For this review, take the finished solid that the model builds, in its own axes (mm). A direction names the side the tool comes from. Round coordinates to 2 decimals unless told otherwise and drop trailing zeros. Loops run counter-clockwise (first coordinate to the right, second up) from the corner with the lowest first, then second, coordinate; pieces in that order, holes last. Notation, with made-up numbers: (51, 4.25) -> (85, 4.25) arc R25 cw to (85, 41.25) -> close; hole circle Ø1 at (15, 88.25). An arc over 180 degrees is marked (long way). One line per question, with ' | ' between items. Start each with the question number.
1. Consider section A-A (y = -130.5). Write out the cut boundary in (x, z), and give its area (3 significant figures).
2. Draft analysis for pull direction Z (two halves, no side actions). For faces 6 (the face through (3, -2, 10)), 7 (the face through (-3, -85, 10)), 8 (the face through (4.848, 8.746, 2.465)), 9 (the face through (0.14, -129.87, 13.09)), state which applies: pulls with the +Z half, pulls with the -Z half, needs draft (parallel to the pull), parting line crosses it, or undercut.
3. For faces 1 (the face through (0, -37, 0)), 2 (the face through (1, -15, 8)), 3 (the face through (-10, -51, 7)), 4 (the face through (5, -85, 7)), 5 (the face through (-5.047, 2, 2)), list the 3-axis set-ups (+Z, -Z, +X, -X, +Y, -Y) from which the entire face can be reached by the end or side of a thin tool; tool diameter is ignored.
4. For pin 1 Ø5.5 at (y, z) = (-200, 8) entering from -X; pin 2 Ø2.5 at (x, z) = (-1.5, 7) entering from +Y; pin 3 Ø4 at (y, z) = (-201, 9) entering from +X; pin 4 Ø2.5 at (x, y) = (0, -85) entering from +Z, all flat-tipped, find the tip position at first contact; note any pin that passes through.
5. Wall thickness on line 1 along Z through (x, y) = (-4.25, -86); line 2 along X through (y, z) = (-85, 11.15); line 3 along X through (y, z) = (-72.5, 7.5): over which ranges is each line inside the solid? List them lowest first.
6. Consider section B-B (y = -158). Write out the cut boundary in (x, z), and give its area (3 significant figures).
```python
from build123d import *

# Parameters (mm, degrees)
CROQUIS1_R              = 1.5
SALIENTE_EXTRUIR1_DEPTH = 15
CROQUIS2_W              = 5
CROQUIS2_H              = 15
CROQUIS2_H_2            = 35
CORTAR_EXTRUIR1_DEPTH   = 60
CROQUIS4_W              = 5
CROQUIS4_H              = 30
CORTAR_EXTRUIR2_DEPTH   = 15
CORTAR_EXTRUIR3_DEPTH   = 40


with BuildPart() as part:
    # Croquis1 → Saliente-Extruir1 (new body)
    with BuildSketch(Plane.XY):
        with BuildLine():
            Line((10, 0), (10, -85))
            Line((10, -85), (2.49701529, -197.5))
            Line((2.49701529, -197.5), (2.49701529, -202.5))
            Line((2.49701529, -202.5), (-2.49701529, -202.5))
            Line((-2.49701529, -202.5), (-2.49701529, -197.5))
            Line((-2.49701529, -197.5), (-10, -85))
            Line((-10, -85), (-10, 0))
            ThreePointArc((-10, 0), (0, 10), (10, 0))
        make_face()
        with Locations((0, -85)):
            Circle(CROQUIS1_R, mode=Mode.SUBTRACT)
        Circle(CROQUIS1_R, mode=Mode.SUBTRACT)
    extrude(amount=SALIENTE_EXTRUIR1_DEPTH)

    # Croquis2 → Cortar-Extruir1 (cut)
    with BuildSketch(Plane(origin=(10, 0, 0), x_dir=(0, 0, -1), z_dir=(1, 0, 0))):
        with Locations((-7.5, -7.5)):
            Rectangle(CROQUIS2_W, CROQUIS2_H)
        with Locations((-7.5, 17.5)):
            Rectangle(CROQUIS2_W, CROQUIS2_H_2)
        Polygon((-15, -85), (-10, -202.5), (-18.081893827, -208.021253548), align=None)
        Polygon((-5, -202.5), (3.081893827, -208.021253548), (0, -85), align=None)
    extrude(amount=-CORTAR_EXTRUIR1_DEPTH, mode=Mode.SUBTRACT)

    # Croquis4 → Cortar-Extruir2 (cut)
    with BuildSketch(Plane.ZY.offset(10)):
        with Locations((7.5, -85)):
            Rectangle(CROQUIS4_W, CROQUIS4_H)
    extrude(amount=-CORTAR_EXTRUIR2_DEPTH, mode=Mode.SUBTRACT)

    # Croquis5 → Cortar-Extruir3 (cut)
    with BuildSketch(Plane(origin=(0, 0, 0), x_dir=(-1, 0, 0), z_dir=(0, 0, -1))):
        with BuildLine():
            Line((20.047011477, -20), (24.874582677, -20))
            Line((24.874582677, -20), (24.874582677, 13.063406197))
            Line((24.874582677, 13.063406197), (10, 13.063406197))
            Line((10, 13.063406197), (10, 14.482732523))
            Line((10, 14.482732523), (5.047011477, 14.482732523))
            Line((5.047011477, 14.482732523), (5.047011477, -5))
            ThreePointArc((5.047011477, -5), (9.440409759, -15.606601718), (20.047011477, -20))
        make_face()
    extrude(amount=-CORTAR_EXTRUIR3_DEPTH, mode=Mode.SUBTRACT)


solid = part.part
```
Answer block:
1) outline: (-6.97, 1.94) -> (6.97, 1.94) -> (6.97, 13.06) -> (-6.97, 13.06) -> close | area: 155 mm2
2) face 6: undercut | face 7: undercut | face 8: needs draft | face 9: pulls with the +Z half
3) face 1: -Z, +X, -X, +Y, -Y | face 2: +X, -X, +Y | face 3: +Z, -Z, -X, +Y, -Y | face 4: -X | face 5: +Z, -Z, -X, +Y
4) pin 1: stops at x = -2.51 | pin 2: stops at y = -15 | pin 3: stops at x = 2.5 | pin 4: passes through
5) line 1: z = 0.04 to 5, 10 to 14.96 | line 2: x = -10 to -1.5, 1.5 to 10 | line 3: x = 5 to 10
6) outline: (-5.13, 3.11) -> (5.13, 3.11) -> (5.13, 11.89) -> (-5.13, 11.89) -> close | area: 90.2 mm2
